Build history of the part. All positions in model axes, mm. Face numbers are marked on the shaded views. A direction names the side the tool comes from. Round coordinates to 2 decimals unless told otherwise and drop trailing zeros. Write each loop counter-clockwise with the first axis right and the second up, starting at its lowest first coordinate (ties: lowest second). Pieces come first, ordered by that corner, then holes.
Item 1: 3-axis set-ups, long thin cutter, end or side, ignore diameter. For the marked faces 1, 2 and 3: which of +Z, -Z, +X, -X, +Y, -Y reach the whole face in a straight line?
Item 2: Band-saw the part on D-D, the plane x = -19. Write the cut outline in (y, z).
Item 3: Drop flat-ended pins along their axis: pin 1 Ø1.2 at (x, y) = (-23.5, 3) entering from -Z; pin 2 Ø1.5 at (x, z) = (-10.5, -4.5) entering from +Y. Give the stop position or say it passes through.
Item 4: Band-saw the part on A-A, the plane z = -5. Write the cut outline in (x, y), then the cut area to 3 significant figures.
Item 5: Mould opens along Z. For the marked faces 4, 5, 6 and 7 say: +Z half, -Z half, draft (parallel to the pull), parting line (faces both ways), or undercut.
Item 6: Band-saw the part on C-C, the plane x = -29. Write the cut outline in (y, z).
Item 7: Wall check: probe 1 along X at (y, z) = (1.9, -5); probe 2 along X at (y, z) = (2.6, -5.75); probe 3 along Y at (x, z) = (-23, -9.25). Give the ranges that are in metal, low to high.
Item 8: Band-saw the part on B-B, the plane y = 1.05. Write the cut outline in (x, z).
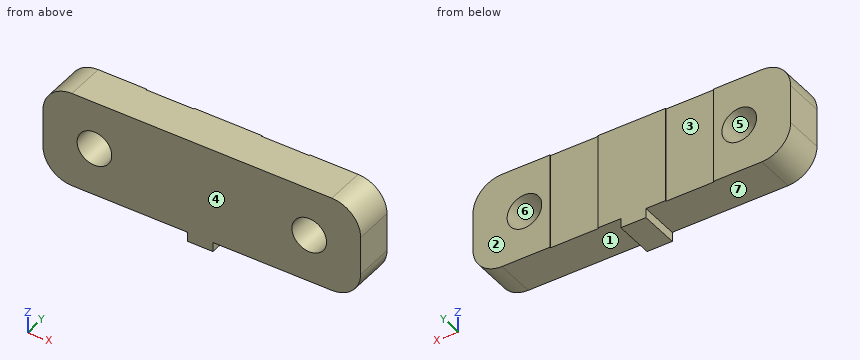
Autodesk Inventor part; units mm, degrees
ref_plane "Work Plane1" through (-16.5, 0, 0) normal (1, 0, 0) x (0, 0, -1)
ref_plane "YZ Plane" through (0, 0, 0) normal (1, 0, 0) x (0, 1, 0)
ref_plane "XZ Plane" through (0, 0, 0) normal (0, 1, 0) x (-1, 0, 0)
sketch "Sketch1" plane through (0, 0, 0) normal (0, 1, 0) x (-1, 0, 0)
  line L0 (0, 0) -> (33, 0)
  line L1 (33, 0) -> (33, -10)
  line L2 (33, -10) -> (0, -10)
  line L3 (0, -10) -> (0, 0)
  dimension "d0" = 33
  dimension "d1" = 10
extrude "Extrusion1" add sketch "Sketch1" along normal blind 4
sketch "Sketch2" plane through (0, 4, 0) normal (0, 1, 0) x (1, 0, 0)
  circle A0 centre (-5.343, 5) radius 1.8
  point P0 (0, 0)
  dimension "d9" = 3.6
extrude "Extrusion2" cut sketch "Sketch2" against normal blind 4
ref_plane "Work Plane1" through (-16.5, 0, 0) normal (1, 0, 0) x (0, 0, -1)
mirror "Mirror1" about plane through (-16.5, 0, 0) normal (1, 0, 0) of "Extrusion2"
fillet "Fillet1" radius 3 4 edges at (-33, 2, 0) (-33, 2, -10) (0, 2, 0) (0, 2, -10)
sketch "Sketch3" plane through (0, 4, 0) normal (0, 1, 0) x (1, 0, 0)
  line L0 (-30, 0) -> (-3, 0)
  line L1 (-30, 10) -> (-3, 10)
  line L2 (-20, 0) -> (-13, 0)
  line L3 (-13, 0) -> (-13, 10)
  line L4 (-13, 10) -> (-20, 10)
  line L5 (-20, 10) -> (-20, 0)
  point P0 (0, 0)
  dimension "d10" = 7
  dimension "d11" = 10
extrude "Extrusion3" add sketch "Sketch3" along normal blind 0.1
sketch "Sketch4" plane through (0, 4, 0) normal (0, 1, 0) x (1, 0, 0)
  line L0 (-3, 0) -> (-8, 0)
  line L1 (-8, 0) -> (-8, 10)
  line L2 (-8, 10) -> (-3, 10)
  line L3 (0, 7) -> (0, 3)
  arc A0 (-3, 0) -> (0, 3) centre (-3, 3) ccw
  arc A1 (0, 7) -> (-3, 10) centre (-3, 7) ccw
  circle A2 centre (-5.343, 5) radius 1.8
  circle A3 centre (-5.343, 5) radius 1.8
  point P0 (0, 0)
  point P1 (0, 10)
  dimension "d14" = 8
  dimension "d15" = 10
  dimension "d16" = 3
extrude "Extrusion4" add sketch "Sketch4" along normal blind 0.1
mirror "Mirror2" about plane through (-16.5, 0, 0) normal (1, 0, 0) of "Extrusion4"
sketch "Sketch6" plane through (0, 4.1, 0) normal (0, 1, 0) x (1, 0, 0)
  line L0 (-15.3522, 9.1051) -> (-17.9653, 9.1051)
  line L1 (-17.9653, 9.1051) -> (-17.9653, 10.9833)
  line L2 (-17.9653, 10.9833) -> (-15.3522, 10.9833)
  line L3 (-15.3522, 10.9833) -> (-15.3522, 9.1051)
  point P0 (0, 0)
extrude "Extrusion6" add sketch "Sketch6" against normal up to surface (4.1 mm away)
properties part number "8 peristaltic pump clamp 0.1mm"
Results:
1. face 1: -Z, +X, +Y, -Y
1. face 2: +Z, -Z, +X, -X, +Y
1. face 3: +Z, -Z, +Y
2. outline: (0, -10) - (4.1, -10) - (4.1, 0) - (0, 0) - close
3. pin 1: stops at z = -10
3. pin 2: stops at y = 4
4. outline: (-33, 0) - (-29.46, 0) - (-29.46, 4.1) - (-33, 4.1) - close; (-25.86, 0) - (-7.14, 0) - (-7.14, 4.1) - (-8, 4.1) - (-8, 4) - (-13, 4) - (-13, 4.1) - (-20, 4.1) - (-20, 4) - (-25, 4) - (-25, 4.1) - (-25.86, 4.1) - close; (-3.54, 0) - (0, 0) - (0, 4.1) - (-3.54, 4.1) - close
4. area: 105 mm2
5. face 4: draft
5. face 5: undercut
5. face 6: undercut
5. face 7: -Z half
6. outline: (0, -10) - (4.1, -10) - (4.1, -6.2) - (0, -6.2) - close; (0, -3.8) - (4.1, -3.8) - (4.1, 0) - (0, 0) - close
7. probe 1: x = -33 to -29.46, -25.86 to -7.14, -3.54 to 0
7. probe 2: x = -33 to -29.29, -26.02 to -6.98, -3.71 to 0
7. probe 3: y = 0 to 4
8. outline: (-33, -7) arc R3 ccw to (-30, -10) - (-17.97, -10) - (-17.97, -10.98) - (-15.35, -10.98) - (-15.35, -10) - (-3, -10) arc R3 ccw to (0, -7) - (0, -3) arc R3 ccw to (-3, 0) - (-30, 0) arc R3 ccw to (-33, -3) - close; hole circle Ø3.6 at (-27.66, -5); hole circle Ø3.6 at (-5.34, -5)
